Can you work these out from the model? Positions are in its coordinate system, mm. A direction names the side the tool comes from. Give positions to 0.01 mm unless a question says otherwise; leave off trailing zeros. Order: outer loops, then holes, each group sorted by start corner. A loop starts at its lowest first (then second) coordinate and runs counter-clockwise, first axis right, second up. Notation, with made-up numbers: (51.25, -19) - (100.25, -19) arc R29 cw to (100.25, 10) - close; hole circle Ø1 at (40, 46.25). An arc over 180 degrees is marked (long way). Use one line per item in the form item = value. Start each with the question number.
1) We'd pull the mould along Y, two halves only. Please class faces 3 (the flat face through (-1, 1, 25.4)), 4 (the cylindrical face through (-13.8, 23.516, 18.961)), 5 (the cylindrical face through (36.59, 11.52, 12.52)): released by +Y, released by -Y, zero draft, split by the parting line, or undercut.
2) Which directions (+Z, -Z, +X, -X, +Y, -Y) give clear straight access to the entire face, cutting with the end or side of a thin tool? Please do faces 1 (the cylindrical face through (17.22, 16.347, 18.961)), 2 (the flat face through (-1, 1, 0)).
3) Suppose I cut it at B-B, the plane z = 9.75. Write out the boundary of the cut face in (x, y).
4) Please list where these lines run through material, in increasing order: probe 1 along Y at (x, z) = (-18.5, 20.75); probe 2 along X at (y, z) = (0.5, 18.5); probe 3 along X at (y, z) = (3, 11.75).
5) Suppose I cut it at D-D, the plane z = 23.25. State how many separate pieces and enclosed holes the cut face has, and give its area (3 significant figures).
6) Suppose I cut it at C-C, the plane x = -22. Write out the boundary of the cut face in (y, z), and give its area (3 significant figures).
7) Suppose I cut it at A-A, the plane y = 0. Write out the boundary of the cut face in (x, z), and give its area (3 significant figures).
8) For pin 1 (1.5 mm diameter, centred on x = 28, z = 19.5, fed in from +Y); pin 2 (6 mm diameter, centred on y = 3.5, z = 19, fed in from +X); pin 3 (12 mm diameter, centred on y = -11.5, z = 4, fed in from +X); pin 4 (6 mm diameter, centred on y = -3, z = 3.5, fed in from -X), each with a flat end and sliding along its axis, tell me the tip position at first contact or that it passes through.
```python
from build123d import *

# Parameters (mm, degrees)
F0_R     = 38.3617531957
F1_DEPTH = 25.4
F2_R     = 7.6146171672
F2_R_2   = 8.1970349446
F3_DEPTH = 25.401
F5_D     = 6.35
F5_DEPTH = 12.7
F5_TIP   = 1.9077324654


with BuildPart() as f1:
    # F0 (on Top) → F1 (new body)
    with BuildSketch(Plane.XY):
        Circle(F0_R)
    extrude(amount=F1_DEPTH)

    # F2 (on face) → F3 (cut, through all)
    with BuildSketch(Plane.XY.offset(25.4)):
        with Locations((16.6444163769, 0)):
            Circle(F2_R)
        with Locations((-18.1044526398, 0)):
            Circle(F2_R_2)
    extrude(amount=-F3_DEPTH, mode=Mode.SUBTRACT)

    # F5
    with Locations(Plane.XY.offset(25.4)):
        with Locations((-16.1400576362, 21.3705980134), (16.5315663715, 19.4467739825)):
            Hole(F5_D / 2, depth=F5_DEPTH)
            with Locations((0, 0, -(F5_DEPTH + F5_TIP / 2))):  # 118° drill point
                Cone(0, F5_D / 2, F5_TIP, mode=Mode.SUBTRACT)


solid = f1.part
```
Result sheet:
q1.face_3 = zero draft
q1.face_4 = undercut
q1.face_5 = split by the parting line
q2.face_1 = +Z
q2.face_2 = -Z, +X, -X, +Y, -Y
q3.outline = circle Ø76.72 at (0, 0); hole circle Ø16.39 at (-18.1, 0); hole circle Ø15.23 at (16.64, 0)
q4.probe_1 = -33.61 to -8.19, 8.19 to 19.25, 23.49 to 33.61
q4.probe_2 = -38.36 to -26.29, -9.92 to 9.05, 24.24 to 38.36
q4.probe_3 = -38.24 to -25.73, -10.48 to 9.65, 23.64 to 38.24
q5.separate_pieces = 1
q5.enclosed_holes = 4
q5.area = 4,170 mm²
q6.outline = (-31.43, 0) - (-7.21, 0) - (-7.21, 25.4) - (-31.43, 25.4) - close; (7.21, 0) - (31.43, 0) - (31.43, 25.4) - (7.21, 25.4) - close
q6.area = 1,230 mm²
q7.outline = (-38.36, 0) - (-26.3, 0) - (-26.3, 25.4) - (-38.36, 25.4) - close; (-9.91, 0) - (9.03, 0) - (9.03, 25.4) - (-9.91, 25.4) - close; (24.26, 0) - (38.36, 0) - (38.36, 25.4) - (24.26, 25.4) - close
q7.area = 1,150 mm²
q8.pin_1 = 27
q8.pin_2 = 38.36
q8.pin_3 = 37.97
q8.pin_4 = -38.36
